Input: part model. Units: mm. Frame: model coordinates. Coordinates: 2 decimals unless noted, no trailing zeros. Order: outer loops, then holes, each group sorted by start corner. A loop starts at its lowest first (then second) coordinate and runs counter-clockwise, first axis right, second up.
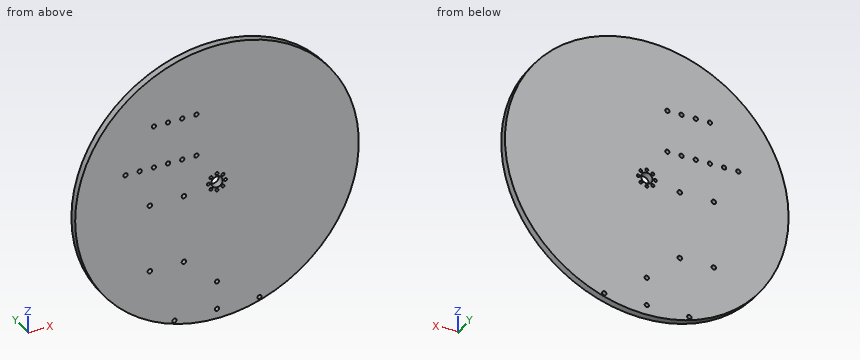
Autodesk Inventor part; units mm, degrees
ref_plane "YZ Plane" through (0, 0, 0) normal (1, 0, 0) x (0, 1, 0)
ref_plane "XZ Plane" through (0, 0, 0) normal (0, 1, 0) x (-1, 0, 0)
ref_plane "XY Plane" through (0, 0, 0) normal (0, 0, 1) x (1, 0, 0)
sketch "スケッチ1" plane through (0, 0, 0) normal (0, 1, 0) x (-1, 0, 0)
  circle A0 centre (0, 0) radius 100
  dimension "d0" = 200
extrude "押し出し1" add sketch "スケッチ1" along normal blind 5
sketch "スケッチ12" plane through (0, 5, 0) normal (0, 1, 0) x (1, 0, 0)
  circle A0 centre (0, 0) radius 100
  circle A1 centre (0, 0) radius 4
  circle A2 centre (0, 0) radius 5
  circle A3 centre (0, 0) radius 6
  circle A4 centre (0, 6) radius 1
  circle A5 centre (-4.2426, 4.2426) radius 1
  circle A6 centre (-6, 0) radius 1
  circle A7 centre (-4.2426, -4.2426) radius 1
  circle A8 centre (0, -6) radius 1
  circle A9 centre (4.2426, -4.2426) radius 1
  circle A10 centre (6, 0) radius 1
  circle A11 centre (4.2426, 4.2426) radius 1
  dimension "d94" = 12
  dimension "d92" = 8
  dimension "d93" = 10
  dimension "d95" = 2
  dimension "d98" = 360
hole "穴5" at (-6, 5, 0) at (-4.2426, 5, 4.2426) at (0, 5, 6) at (0, 5, -6) at (4.2426, 5, -4.2426) at (6, 5, 0) at (4.2426, 5, 4.2426) at (-4.2426, 5, -4.2426) direction (0, -1, 0) diameter 2.1 depth 8 tip angle 118
sketch "スケッチ13" plane through (0, 5, 0) normal (0, 1, 0) x (1, 0, 0)
  circle A0 centre (0, 0) radius 100
  circle A1 centre (0, 0) radius 4
  dimension "d107" = 8
extrude "押し出し4" cut sketch "スケッチ13" against normal blind 8 contours A1
sketch "スケッチ14" plane through (0, 5, 0) normal (0, 1, 0) x (1, 0, 0)
  circle A0 centre (0, 0) radius 100
  line L0 (0, 0) -> (0, 63)
  line L1 (0, 63) -> (0, 73)
  line L2 (0, 73) -> (0, 93)
  line L3 (0, 73) -> (30, 73)
  line L4 (0, 73) -> (-30, 73)
  line L5 (-30, 73) -> (30, 73)
  line L6 (30, 73) -> (30, 93)
  line L7 (30, 93) -> (-30, 93)
  line L8 (-30, 93) -> (-30, 73)
  line L9 (0, 0) -> (0, -38.43)
  line L10 (0, -38.43) -> (-14.5, -38.43)
  line L11 (-14.5, -38.43) -> (-14.5, -23.43)
  line L12 (-14.5, -23.43) -> (-24.5, -23.43)
  line L13 (-24.5, -23.43) -> (-34.5, -23.43)
  line L14 (-34.5, -23.43) -> (-44.5, -23.43)
  line L15 (-44.5, -23.43) -> (-54.5, -23.43)
  line L16 (-54.5, -23.43) -> (-64.5, -23.43)
  line L17 (-24.5, -53.43) -> (-34.5, -53.43)
  line L18 (-34.5, -53.43) -> (-44.5, -53.43)
  line L19 (-44.5, -53.43) -> (-54.5, -53.43)
  line L20 (-54.5, -53.43) -> (-64.5, -53.43)
  point P0 (-14.5, -53.43)
  point P1 (-7.25, -38.43)
  dimension "d110" = 63
  dimension "d111" = 10
  dimension "d112" = 20
  dimension "d114" = 30
  dimension "d115" = 30
  dimension "d117" = 14.5
  dimension "d118" = 15
  dimension "d119" = 10
  dimension "d120" = 10
  dimension "d121" = 10
  dimension "d122" = 10
  dimension "d123" = 10
  dimension "d143" = 111.43
hole "穴6" at (-30, 5, -93) at (-30, 5, -73) at (0, 5, -93) at (0, 5, -73) at (30, 5, -73) at (30, 5, -93) at (-64.5, 5, 23.43) at (-54.5, 5, 23.43) at (-44.5, 5, 23.43) at (-34.5, 5, 23.43) at (-24.5, 5, 23.43) at (-14.5, 5, 23.43) at (-64.5, 5, 53.43) at (-54.5, 5, 53.43) at (-44.5, 5, 53.43) at (-34.5, 5, 53.43) at (-24.5, 5, 53.43) at (-14.5, 5, 53.43) at (-30, 5, -93) at (-30, 5, -73) direction (0, -1, 0) diameter 3 depth 8 tip angle 118
sketch "スケッチ16" plane through (0, 5, 0) normal (0, 1, 0) x (1, 0, 0)
  circle A0 centre (-64.5, -53.43) radius 1.5
  circle A1 centre (30, 73) radius 1.5
  circle A2 centre (-30, 73) radius 1.5
  circle A3 centre (-54.5, -53.43) radius 1.5
  circle A4 centre (0, 0) radius 100
  circle A5 centre (0, 0) radius 78
  circle A6 centre (0, 0) radius 90
  circle A7 centre (-54.5, -53.43) radius 1.5
  circle A8 centre (-64.5, -53.43) radius 1.5
  circle A9 centre (-30, 73) radius 1.5
  circle A10 centre (30, 73) radius 1.5
  dimension "d145" = 156
  dimension "d147" = 180
extrude "押し出し7" add sketch "スケッチ16" against normal blind 5 contours A0 | A1 A5 | A5 A1 | A5 A2 | A2 A5 | A3
sketch "スケッチ17" plane through (0, 0, 0) normal (0, -1, 0) x (1, 0, 0)
  line L0 (-50.2739, -0.7823) -> (-20.2739, -0.7823)
  line L1 (-20.2739, -0.7823) -> (-20.2739, -54.7823)
  line L2 (-20.2739, -54.7823) -> (-50.2739, -54.7823)
  line L3 (-50.2739, -54.7823) -> (-50.2739, -0.7823)
  point P0 (-47.2739, -3.7823)
  point P1 (-47.2739, -51.7823)
  point P2 (-23.2739, -51.7823)
  point P3 (-23.2739, -3.7823)
  dimension "d150" = 30
  dimension "d151" = 54
  dimension "d153" = 3
  dimension "d154" = 48
  dimension "d155" = 3
  dimension "d156" = 3
  dimension "d157" = 24
  dimension "d158" = 24
  dimension "d159" = 3
  dimension "d160" = 48
hole "穴7" at (-47.2739, 0, -3.7823) at (-47.2739, 0, -51.7823) at (-23.2739, 0, -51.7823) at (-23.2739, 0, -3.7823) direction (0, 1, 0) diameter 3.2 depth 8 tip angle 118
properties part number "知能ロボコンターンテーブル1.1" material "アセタール樹脂、白"
Item 1: Cut plane A-A on y = 1.8. Count the separate pieces of the cut face and the enclosed holes in it, then the cut area to 3 significant figures.
Response values:
separate pieces: 1
enclosed holes: 27
area: 31,200 mm2
Item 2: Ray query, probe 1 along Z at (x, y) = (-35.5, 0.85); probe 2 along Z at (x, y) = (-14.5, 3.1); probe 3 along X at (y, z) = (1.95, -93). Return the intervals inside material, ascending.
Response values:
probe 1: z = -93.49 to 22.31, 24.55 to 52.31, 54.55 to 93.49
probe 2: z = -98.94 to 21.93, 24.93 to 51.93, 54.93 to 98.94
probe 3: x = -36.76 to -31.5, -28.5 to -1.5, 1.5 to 28.5, 31.5 to 36.76
Item 3: Cut plane C-C on x = 86.5. Return loops of the section in (y, z).
Response values:
outline: (0, -50.18) - (5, -50.18) - (5, 50.18) - (0, 50.18) - close
Item 4: Cut plane B-B on z = -33. Return loops of the section in (x, y).
Response values:
outline: (-94.4, 0) - (94.4, 0) - (94.4, 5) - (-94.4, 5) - close
Item 5: Pin query (flat end, axial travel): pin 1 Ø1 at (x, y) = (-22.5, 2.5) entering from +Z; pin 2 Ø3 at (y, z) = (0.5, -24) entering from -X; pin 3 Ø2.5 at (x, z) = (-54.5, 23.43) entering from +Y; pin 4 Ø2 at (y, z) = (2.5, 33) entering from +X. Return the tip coordinate at first contact, or that it passes through.
Response values:
pin 1: stops at z = 97.55
pin 2: stops at x = -97.44
pin 3: passes through
pin 4: stops at x = 94.74
